Build history of the part. All positions in model axes, mm. Round coordinates to 2 decimals unless told otherwise and drop trailing zeros. Loops run counter-clockwise (first coordinate to the right, second up) from the corner with the lowest first, then second, coordinate; pieces in that order, holes last. Notation, with made-up numbers: (9, 60) - (32, 60) arc R25 ccw to (32, 92) - close; hole circle Ø11 at (-34.75, 10). An arc over 180 degrees is marked (long way). One line per question, with ' | ' between items. Start each with the question number.
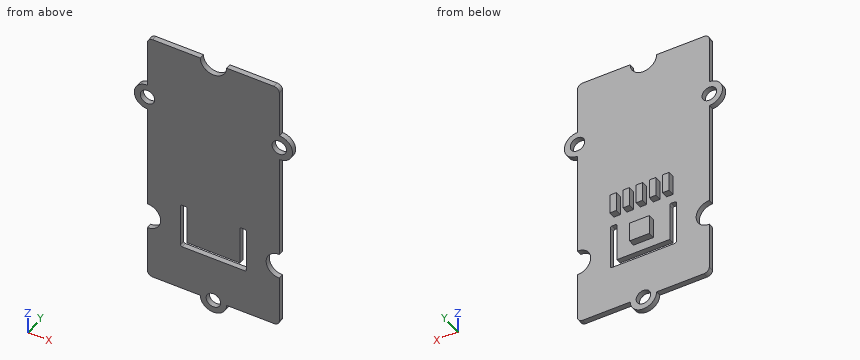
from build123d import *

# Parameters (mm, degrees)
SKETCH1_R        = 1.1
BOARD_DEPTH      = 0.8
U_CUT_DEPTH      = 48.419827077
U_CUT_DEPTH_BACK = 48.419827077
SKETCH3_W        = 1
SKETCH3_H        = 3
SKETCH3_W_2      = 3
SMDS_DEPTH       = 1


with BuildPart() as part:
    # Sketch1 → Board (new body)
    with BuildSketch(Plane(origin=(0, 0, 0), x_dir=(1, 0, 0), z_dir=(0, 1, 0))):
        with BuildLine():
            Line((0.8, 0), (8, 0))
            ThreePointArc((8, 0), (10, 2), (12, 0))
            Line((12, 0), (19.2, 0))
            ThreePointArc((19.2, 0), (19.765685425, 0.234314575), (20, 0.8))
            Line((20, 0.8), (20, 8))
            ThreePointArc((20, 8), (22, 10), (20, 12))
            Line((20, 12), (20, 28))
            ThreePointArc((20, 28), (18, 30), (20, 32))
            Line((20, 32), (20, 39.2))
            ThreePointArc((20, 39.2), (19.765685425, 39.765685425), (19.2, 40))
            Line((19.2, 40), (12, 40))
            ThreePointArc((12, 40), (10, 42), (8, 40))
            Line((8, 40), (0.8, 40))
            ThreePointArc((0.8, 40), (0.234314575, 39.765685425), (0, 39.2))
            Line((0, 39.2), (0, 32))
            ThreePointArc((0, 32), (2, 30), (0, 28))
            Line((0, 28), (0, 12))
            ThreePointArc((0, 12), (-2, 10), (0, 8))
            Line((0, 8), (0, 0.8))
            ThreePointArc((0, 0.8), (0.234314575, 0.234314575), (0.8, 0))
        make_face()
        with Locations(Location((10, 40, 0), (0, 0, 270))):
            Circle(SKETCH1_R, mode=Mode.SUBTRACT)
        with Locations(Location((0, 10, 0), (0, 0, 270))):
            Circle(SKETCH1_R, mode=Mode.SUBTRACT)
        with Locations(Location((20, 10, 0), (0, 0, 270))):
            Circle(SKETCH1_R, mode=Mode.SUBTRACT)
    extrude(amount=BOARD_DEPTH)

    # Sketch2 → U-cut (cut, two sides: drawn at the far end of the back side and taken through both)
    with BuildSketch(Plane(origin=(0, 0.8, 0), x_dir=(1, 0, 0), z_dir=(0, 1, 0)).offset(-U_CUT_DEPTH_BACK)):
        with BuildLine():
            Line((14.25, 26), (14.75, 26))
            ThreePointArc((14.75, 26), (14.926776695, 26.073223305), (15, 26.25))
            Line((15, 26.25), (15, 32.75))
            ThreePointArc((15, 32.75), (14.926776695, 32.926776695), (14.75, 33))
            Line((14.75, 33), (5.25, 33))
            ThreePointArc((5.25, 33), (5.073223305, 32.926776695), (5, 32.75))
            Line((5, 32.75), (5, 26.25))
            ThreePointArc((5, 26.25), (5.073223305, 26.073223305), (5.25, 26))
            Line((5.25, 26), (5.75, 26))
            ThreePointArc((5.75, 26), (5.926776695, 26.073223305), (6, 26.25))
            Line((6, 26.25), (6, 32))
            Line((6, 32), (14, 32))
            Line((14, 32), (14, 26.25))
            ThreePointArc((14, 26.25), (14.073223305, 26.073223305), (14.25, 26))
        make_face()
    extrude(amount=U_CUT_DEPTH + U_CUT_DEPTH_BACK, mode=Mode.SUBTRACT)

    # Sketch3 → SMDs (add)
    with BuildSketch(Plane(origin=(0, 0.8, 0), x_dir=(1, 0, 0), z_dir=(0, 1, 0))):
        with Locations((6, 23.125)):
            Rectangle(SKETCH3_W, SKETCH3_H)
        with Locations((8, 23.125)):
            Rectangle(SKETCH3_W, SKETCH3_H)
        with Locations((10, 23.125)):
            Rectangle(SKETCH3_W, SKETCH3_H)
        with Locations((12, 23.125)):
            Rectangle(SKETCH3_W, SKETCH3_H)
        with Locations((14, 23.125)):
            Rectangle(SKETCH3_W, SKETCH3_H)
        with Locations((10, 29.125)):
            Rectangle(SKETCH3_W_2, SKETCH3_H)
    extrude(amount=SMDS_DEPTH)


solid = part.part
1) Drop flat-ended pins along their axis: pin 1 (0.9 mm diameter, centred on y = 0.5, z = -4.5, fed in from -X); pin 2 (0.6 mm diameter, centred on y = 0.5, z = -37, fed in from +X); pin 3 (0.6 mm diameter, centred on x = 5.5, y = 0.5, fed in from -Z); pin 4 (2 mm diameter, centred on x = 0, z = -10, fed in from +Y). Give the stop position or say it passes through.
2) Saw through at A-A on y = 1.4. Write the cut outline in (x, z) (3 decimals), and give its area (3 significant figures).
3) Wall check: line 1 (X direction, y = 0.55, z = -10); line 2 (X direction, y = 0.35, z = -27.5); line 3 (Y direction, x = 17.25, z = -8). Give the ranges that are in metal, low to high. Write a range as [from, to].
4) Saw through at C-C on x = 10. Write the cut outline in (y, z) (3 decimals), and give its area (3 significant figures).
5) Saw through at B-B on z = -30. Write the cut outline in (x, y).
6) Saw through at D-D on z = -10. Write the cut outline in (x, y).
Answer key:
1) pin 1: x = 0 | pin 2: x = 20 | pin 3: z = -40 | pin 4: through
2) outline: (5.5, -24.625) - (6.5, -24.625) - (6.5, -21.625) - (5.5, -21.625) - close; (7.5, -24.625) - (8.5, -24.625) - (8.5, -21.625) - (7.5, -21.625) - close; (8.5, -30.625) - (11.5, -30.625) - (11.5, -27.625) - (8.5, -27.625) - close; (9.5, -24.625) - (10.5, -24.625) - (10.5, -21.625) - (9.5, -21.625) - close; (11.5, -24.625) - (12.5, -24.625) - (12.5, -21.625) - (11.5, -21.625) - close; (13.5, -24.625) - (14.5, -24.625) - (14.5, -21.625) - (13.5, -21.625) - close | area: 24.0 mm²
3) line 1: [-2, -1.1], [1.1, 18.9], [21.1, 22] | line 2: [0, 5], [6, 14], [15, 20] | line 3: [0, 0.8]
4) outline: (0, -42) - (0.8, -42) - (0.8, -41.1) - (0, -41.1) - close; (0, -38.9) - (0.8, -38.9) - (0.8, -33) - (0, -33) - close; (0, -32) - (0.8, -32) - (0.8, -30.625) - (1.8, -30.625) - (1.8, -27.625) - (0.8, -27.625) - (0.8, -24.625) - (1.8, -24.625) - (1.8, -21.625) - (0.8, -21.625) - (0.8, -2) - (0, -2) - close | area: 35.4 mm²
5) outline: (2, 0) - (5, 0) - (5, 0.8) - (2, 0.8) - close; (6, 0) - (14, 0) - (14, 0.8) - (11.5, 0.8) - (11.5, 1.8) - (8.5, 1.8) - (8.5, 0.8) - (6, 0.8) - close; (15, 0) - (18, 0) - (18, 0.8) - (15, 0.8) - close
6) outline: (-2, 0) - (-1.1, 0) - (-1.1, 0.8) - (-2, 0.8) - close; (1.1, 0) - (18.9, 0) - (18.9, 0.8) - (1.1, 0.8) - close; (21.1, 0) - (22, 0) - (22, 0.8) - (21.1, 0.8) - close
